CAD build for the part. Positions are in the model's coordinates, mm. Face numbers are marked on the shaded views. A direction names the side the tool comes from. Round coordinates to 2 decimals unless told otherwise and drop trailing zeros. Loops run counter-clockwise (first coordinate to the right, second up) from the corner with the lowest first, then second, coordinate; pieces in that order, holes last. Notation, with made-up numbers: (-21, 38.25) -> (32, 38.25) arc R5 cw to (32, 46.25) -> close; hole circle Ø7 at (46.25, 20.25). An arc over 180 degrees is marked (long way). Answer as CSV lines item,"result".
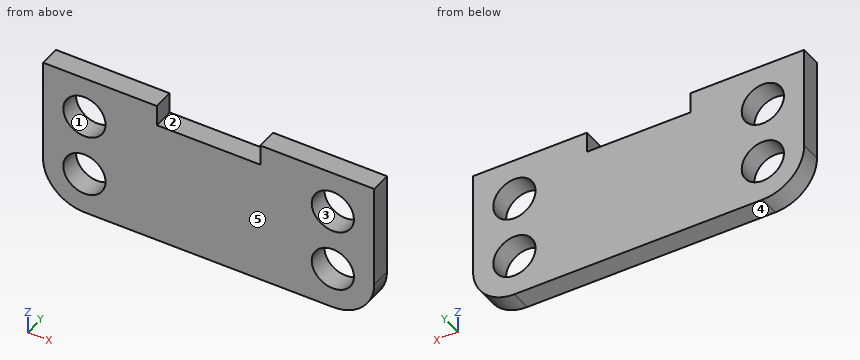
```python
from build123d import *

# Parameters (mm, degrees)
SKETCH1_R           = 6.477
BOSS_EXTRUDE1_DEPTH = 3.175


with BuildPart() as part:
    # Sketch1 → Boss-Extrude1 (new, symmetric)
    with BuildSketch(Plane(origin=(0, 0, 0), x_dir=(1, 0, 0), z_dir=(0, 1, 0))):
        with BuildLine():
            Line((38.1, 38.1), (-38.1, 38.1))
            ThreePointArc((-38.1, 38.1), (-47.080256121, 34.380256121), (-50.8, 25.4))
            Line((-50.8, 25.4), (-50.8, -6.35))
            Line((-50.8, -6.35), (-15.875, -6.35))
            Line((-15.875, -6.35), (-15.875, 0))
            Line((-15.875, 0), (15.875, 0))
            Line((15.875, 0), (15.875, -6.35))
            Line((15.875, -6.35), (50.8, -6.35))
            Line((50.8, -6.35), (50.8, 25.4))
            ThreePointArc((50.8, 25.4), (47.080256121, 34.380256121), (38.1, 38.1))
        make_face()
        with Locations(Location((-38.1, 25.4, 0), (0, 0, 270))):
            Circle(SKETCH1_R, mode=Mode.SUBTRACT)
        with Locations(Location((-38.1, 6.35, 0), (0, 0, 270))):
            Circle(SKETCH1_R, mode=Mode.SUBTRACT)
        with Locations(Location((38.1, 25.4, 0), (0, 0, 270))):
            Circle(SKETCH1_R, mode=Mode.SUBTRACT)
        with Locations(Location((38.1, 6.35, 0), (0, 0, 270))):
            Circle(SKETCH1_R, mode=Mode.SUBTRACT)
    extrude(amount=BOSS_EXTRUDE1_DEPTH, both=True)


solid = part.part
```
Q1. Probe L1, parallel to X at y = 1.75, z = -6.35; L2, parallel to X at y = 2.75, z = -8.5; L3, parallel to Z at x = -13, y = -2. List the from-to ranges inside material, lowest first. Write a range as [from, to].
Results:
L1,"[-50.8, -44.58], [-31.62, 31.62], [44.58, 50.8]"
L2,"[-50.8, -44.21], [-31.99, 31.99], [44.21, 50.8]"
L3,"[-38.1, 0]"
Q2. Slice it at B-B, the plane z = -5. Give the cut face in (x, y) (3 decimals).
Results:
outline,"(-50.8, -3.175) -> (-44.435, -3.175) -> (-44.435, 3.175) -> (-50.8, 3.175) -> close; (-31.765, -3.175) -> (31.765, -3.175) -> (31.765, 3.175) -> (-31.765, 3.175) -> close; (44.435, -3.175) -> (50.8, -3.175) -> (50.8, 3.175) -> (44.435, 3.175) -> close"
Q3. Two-plate mould, pull along Z, no slides. Class the marked faces 3, 4 and 5: pulls with the +Z half, pulls with the -Z half, needs draft (parallel to the pull), parting line crosses it, or undercut.
Results:
face 3,"undercut"
face 4,"pulls with the -Z half"
face 5,"needs draft"
Q4. Slice it at D-D, the plane x = 1.5. Give the cut face in (y, z) (3 decimals).
Results:
outline,"(-3.175, -38.1) -> (3.175, -38.1) -> (3.175, 0) -> (-3.175, 0) -> close"
Q5. Drop flat-ended pins along their axis: pin 1 Ø3 at (y, z) = (-2, -28) entering from +X; pin 2 Ø3 at (x, y) = (0.5, -0.5) entering from +Z. Give the stop position or say it passes through.
Results:
pin 1,"x = 50.75"
pin 2,"z = 0"
Q6. Tool access for the marked faces 1 and 2: list every direction of +Z, -Z, +X, -X, +Y, -Y with a clear straight run to the whole face (end or side of a thin tool).
Results:
face 1,"+Y, -Y"
face 2,"+Z, +Y, -Y"
Q7. Slice it at A-A, the plane y = -0.75. Give the cut face in (x, z) (3 decimals), and give its area (3 significant figures).
Results:
outline,"(-50.8, -25.4) arc R12.7 ccw to (-38.1, -38.1) -> (38.1, -38.1) arc R12.7 ccw to (50.8, -25.4) -> (50.8, 6.35) -> (15.875, 6.35) -> (15.875, 0) -> (-15.875, 0) -> (-15.875, 6.35) -> (-50.8, 6.35) -> close; hole circle Ø12.954 at (-38.1, -25.4); hole circle Ø12.954 at (-38.1, -6.35); hole circle Ø12.954 at (38.1, -25.4); hole circle Ø12.954 at (38.1, -6.35)"
area,"3,720 mm2"
Q8. Slice it at C-C, the plane x = -40. Give the cut face in (y, z) (3 decimals).
Results:
outline,"(-3.175, -37.957) -> (3.175, -37.957) -> (3.175, -31.592) -> (-3.175, -31.592) -> close; (-3.175, -19.208) -> (3.175, -19.208) -> (3.175, -12.542) -> (-3.175, -12.542) -> close; (-3.175, -0.158) -> (3.175, -0.158) -> (3.175, 6.35) -> (-3.175, 6.35) -> close"
